Geometry: see drawing. Coordinates: mm, zero at the bounding-box minimum. A direction names the side the tool comes from. Round coordinates to 2 decimals unless told otherwise and drop trailing zeros. Write each loop counter-clockwise with the first axis right and the second up, starting at its lowest first coordinate (ties: lowest second). Pieces come first, ordered by that corner, then holes. Notation, with made-up numbers: M -26,-30 L 23,-30 A19 ccw 23,-22 Z; hole C 1.5,50 d7. An arc over 180 degrees is marked long. Use one line per item in the form item = value. Start each with the question number.
Item 1: Section query B-B (x = 17.25). Return loops of the section in (y, z) (3 decimals).
Item 2: Pin query (flat end, axial travel): pin 1 Ø10 at (x, y) = (15.5, 15.5) entering from +Z; pin 2 Ø1 at (x, z) = (9, 31.5) entering from +Y; pin 3 Ø3.5 at (x, y) = (3.75, 17.75) entering from +Z; pin 4 Ø7.5 at (x, y) = (4, 18) entering from +Z. Return the tip coordinate at first contact, or that it passes through.
Item 3: Section query C-C (z = 33). Return loops of the section in (x, y) (3 decimals), and give its area (3 significant figures).
Item 4: Pull-direction query (X, two-part tool) for the marked faces 1, 2 and 3; classes: pulls with the +X half, pulls with the -X half, needs draft (parallel to the pull), parting line crosses it, or undercut.
Item 5: Reachability of the marked faces 4, 5 and 6 from +Z, -Z, +X, -X, +Y, -Y: full face, straight path, thin tool, end or side. Return the list, or none.
Item 6: Section query A-A (y = 7.75). Return loops of the section in (x, z) (3 decimals).
Item 7: Ray query, probe 1 along Y at (x, z) = (51.75, 26.75) (3 decimals); probe 2 along Z at (x, y) = (49.5, 20.75); probe 3 along X at (y, z) = (11.25, 31.5). Return the intervals inside material, ascending.
Item 8: Section query D-D (y = 4). Return loops of the section in (x, z).
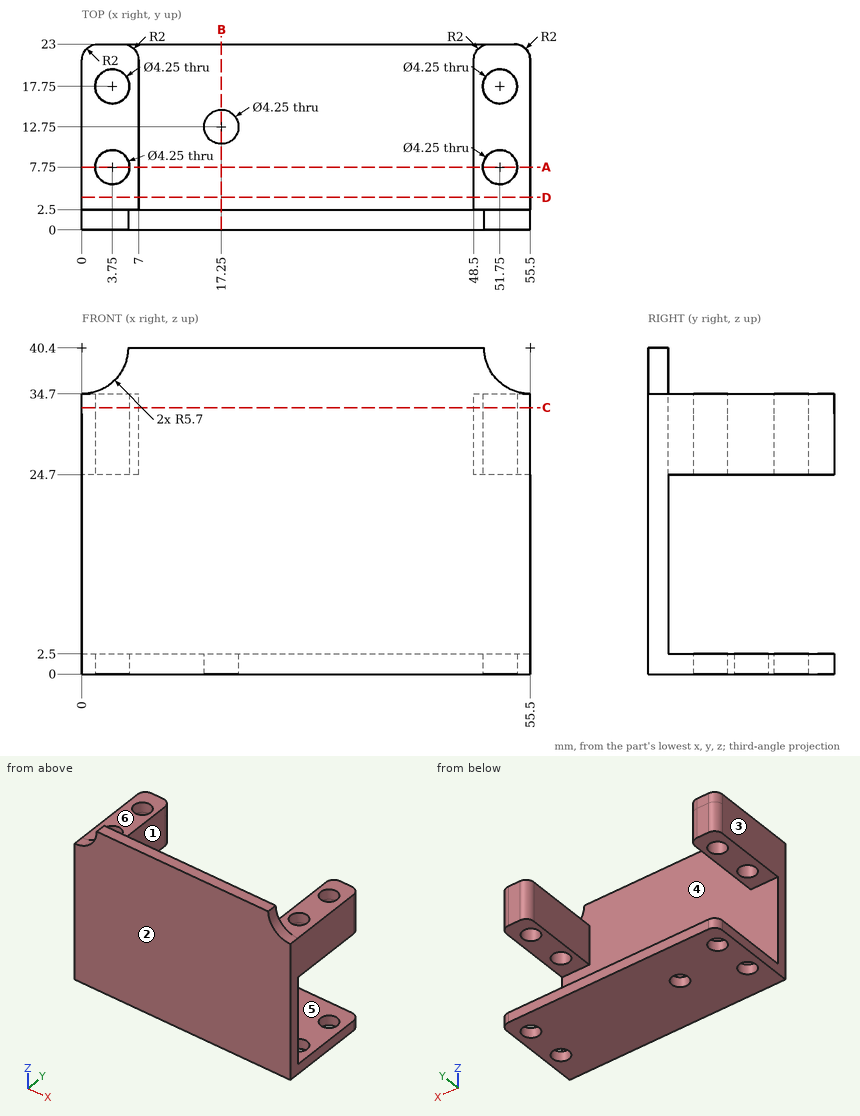
Working result:
q1.outline = M 0,0 L 10.625,0 L 10.625,2.5 L 2.5,2.5 L 2.5,40.4 L 0,40.4 Z; M 14.875,0 L 23,0 L 23,2.5 L 14.875,2.5 Z
q2.pin_1 = 2.5
q2.pin_2 = 2.5
q2.pin_3 = through
q2.pin_4 = 34.7
q3.outline = M 0,0 L 55.5,0 L 55.5,21 A2 ccw 53.5,23 L 50.5,23 A2 ccw 48.5,21 L 48.5,2.5 L 7,2.5 L 7,21 A2 ccw 5,23 L 2,23 A2 ccw 0,21 Z; hole C 3.75,7.75 d4.25; hole C 3.75,17.75 d4.25; hole C 51.75,7.75 d4.25; hole C 51.75,17.75 d4.25
q3.area = 366 mm²
q4.face_1 = undercut
q4.face_2 = needs draft
q4.face_3 = pulls with the -X half
q5.face_4 = +Y
q5.face_5 = +X, -X, +Y
q5.face_6 = +Z, +X, -X, +Y
q6.outline = M 0,0 L 1.625,0 L 1.625,2.5 L 0,2.5 Z; M 0,24.7 L 1.625,24.7 L 1.625,34.7 L 0,34.7 Z; M 5.875,0 L 49.625,0 L 49.625,2.5 L 5.875,2.5 Z; M 5.875,24.7 L 7,24.7 L 7,34.7 L 5.875,34.7 Z; M 48.5,24.7 L 49.625,24.7 L 49.625,34.7 L 48.5,34.7 Z; M 53.875,0 L 55.5,0 L 55.5,2.5 L 53.875,2.5 Z; M 53.875,24.7 L 55.5,24.7 L 55.5,34.7 L 53.875,34.7 Z
q7.probe_1 = 0 to 5.625, 9.875 to 15.625, 19.875 to 23
q7.probe_2 = 0 to 2.5, 24.7 to 34.7
q7.probe_3 = 0 to 7, 48.5 to 55.5
q8.outline = M 0,0 L 55.5,0 L 55.5,2.5 L 0,2.5 Z; M 0,24.7 L 7,24.7 L 7,34.7 L 0,34.7 Z; M 48.5,24.7 L 55.5,24.7 L 55.5,34.7 L 48.5,34.7 Z
